```python
from build123d import *

# Parameters (mm, degrees)
SKETCH1_R           = 40.564550707
BOSS_EXTRUDE1_DEPTH = 10
BOSS_EXTRUDE2_DEPTH = 5.38
SKETCH5_R           = 76.2
BOSS_EXTRUDE3_DEPTH = 5.583348686
BOSS_EXTRUDE4_START = 9.66
SKETCH5_2_R         = 76.2
BOSS_EXTRUDE4_DEPTH = 9.66


with BuildPart() as part:
    # Sketch1 → Boss-Extrude1 (new body)
    with BuildSketch(Plane.XY):
        Circle(SKETCH1_R)
    extrude(amount=BOSS_EXTRUDE1_DEPTH)

    # Sketch2 → Boss-Extrude2 (add)
    with BuildSketch(Plane(origin=(0, 0, 0), x_dir=(-1, 0, 0), z_dir=(0, 0, -1))):
        with BuildLine():
            ThreePointArc((18.605098838, 17.572080057), (25.140246466, 15.180270653), (24.214003726, 8.283098686))
            ThreePointArc((24.214003726, 8.283098686), (25.586626057, 0.502262214), (24.520417146, -7.326448205))
            ThreePointArc((24.520417146, -7.326448205), (25.716623254, -14.181956771), (19.280375747, -16.828393011))
            ThreePointArc((19.280375747, -16.828393011), (13.228284865, -21.907537055), (5.915318308, -24.898528262))
            ThreePointArc((5.915318308, -24.898528262), (0.576376788, -29.362227423), (-4.933627979, -25.111491697))
            ThreePointArc((-4.933627979, -25.111491697), (-12.358341192, -22.409799269), (-18.605098838, -17.572080057))
            ThreePointArc((-18.605098838, -17.572080057), (-25.140246466, -15.180270653), (-24.214003726, -8.283098686))
            ThreePointArc((-24.214003726, -8.283098686), (-25.586626057, -0.502262214), (-24.520417146, 7.326448205))
            ThreePointArc((-24.520417146, 7.326448205), (-25.716623254, 14.181956771), (-19.280375747, 16.828393011))
            ThreePointArc((-19.280375747, 16.828393011), (-13.228284865, 21.907537055), (-5.915318308, 24.898528262))
            ThreePointArc((-5.915318308, 24.898528262), (-0.576376788, 29.362227423), (4.933627979, 25.111491697))
            ThreePointArc((4.933627979, 25.111491697), (12.358341192, 22.409799269), (18.605098838, 17.572080057))
        make_face()
    extrude(amount=BOSS_EXTRUDE2_DEPTH)

    # Sketch4 → Cut-Revolve2 (revolve, cut)
    with BuildSketch(Plane(origin=(0, 0, 0), x_dir=(0, 0, -1), z_dir=(0.9998069773781536, -0.01964708594067849, 0)), mode=Mode.PRIVATE) as cut_revolve2_sk:
        Polygon((0.153479633, 36.092584483), (0.153479633, 40.603125703), (-4.416651314, 40.603125703), (-4.416651314, 35.514398024), (-3.556, 32.394803966), (-3.556, 29.327755228), (0.657751111, 29.301116836), align=None)
    revolve(cut_revolve2_sk.sketch.rotate(Axis((0, 0, 95.775716375), (0, 0, -1)), 178.874232462), axis=Axis((0, 0, 95.775716375), (0, 0, -1)), mode=Mode.SUBTRACT)

    # Sketch5 → Boss-Extrude3 (add)
    with BuildSketch(Plane.XY.offset(10)):
        Circle(SKETCH5_R)
    extrude(amount=-BOSS_EXTRUDE3_DEPTH)

    # Sketch5<2> → Boss-Extrude4 (add)
    with BuildSketch(Plane.XY.offset(10).offset(BOSS_EXTRUDE4_START)):
        Circle(SKETCH5_2_R)
    extrude(amount=-BOSS_EXTRUDE4_DEPTH)


solid = part.part
```
Can you work these out from the model? Positions are in its coordinate system, mm. A direction names the side the tool comes from. Round coordinates to 2 decimals unless told otherwise and drop trailing zeros. Loops run counter-clockwise (first coordinate to the right, second up) from the corner with the lowest first, then second, coordinate; pieces in that order, holes last.
Item 1: Suppose I cut it at B-B, the plane x = 52. Write out the boundary of the cut face in (y, z), then the cut area to 3 significant figures.
Item 2: Suppose I cut it at C-C, the plane y = -51.5. Write out the boundary of the cut face in (x, z), then the cut area to 3 significant figures.
Item 3: Please list where these lines run through material, in increasing order: L1, parallel to Z at x = 11.5, y = -43; L2, parallel to X at y = -12, z = -0.75; L3, parallel to X at y = -16.5, z = 0.25.
Item 4: Suppose I cut it at A-A, the plane z = -2.5. Write out the boundary of the cut face in (x, y).
Item 5: Suppose I cut it at D-D, the plane z = 13.25. Write out the boundary of the cut face in (x, y), then the cut area to 3 significant figures.
Item 6: Which directions (+Z, -Z, +X, -X, +Y, -Y) give clear straight access to the entire face, cutting with the end or side of a thin tool? Please do faces 1 (the cylindrical face through (0.68, 29.36, -2.65)), 2 (the conical face through (28.62, 6.35, 1.42)), 3 (the cylindrical face through (-25.584, 0.613, -2.652)), 4 (the cylindrical face through (-0.68, -29.36, -2.65)).
Item 7: If we mould it in two halves opening along Y, with no side actions, what happens to faces 5 (the flat face through (-13, 24, 0)), 6 (the cylindrical face through (25.584, -0.613, -2.652)), 7 (the cylindrical face through (-25.085, 15.27, -2.652)), 8 (the conical face through (-32.27, 4.24, 3.6))? For each: +Y half, -Y half, draft (parallel to the pull), parting line (faces both ways), or undercut.
Item 8: Will these pins go through, and if not, where does the flat tip stop? pin 1 Ø1.5 at (x, z) = (-42.5, 5) entering from -Y; pin 2 Ø1.5 at (x, z) = (-26, 9.5) entering from +Y; pin 3 Ø8 at (x, y) = (-61, 38) entering from -Z.
Reported:
1. outline: (-55.7, 4.42) - (55.7, 4.42) - (55.7, 19.66) - (-55.7, 19.66) - close
1. area: 1,700 mm2
2. outline: (-56.16, 4.42) - (56.16, 4.42) - (56.16, 19.66) - (-56.16, 19.66) - close
2. area: 1,710 mm2
3. L1: z = 4.42 to 19.66
3. L2: x = -26.38 to 25.93
3. L3: x = -24.22 to 24.22
4. outline: (-24.52, -7.33) arc R5.56 ccw to (-19.28, -16.83) arc R25.59 ccw to (-5.92, -24.9) arc R5.56 ccw to (4.93, -25.11) arc R25.59 ccw to (18.61, -17.57) arc R5.56 ccw to (24.21, -8.28) arc R25.59 ccw to (24.52, 7.33) arc R5.56 ccw to (19.28, 16.83) arc R25.59 ccw to (5.92, 24.9) arc R5.56 ccw to (-4.93, 25.11) arc R25.59 ccw to (-18.61, 17.57) arc R5.56 ccw to (-24.21, 8.28) arc R25.59 ccw to start
5. outline: circle Ø152.4 at (0, 0)
5. area: 18,200 mm2
6. face 1: -Z, +Y
6. face 2: -Z
6. face 3: -Z, -X
6. face 4: -Z, -Y
7. face 5: draft
7. face 6: undercut
7. face 7: undercut
7. face 8: parting line
8. pin 1: stops at y = -63.74
8. pin 2: stops at y = 71.89
8. pin 3: stops at z = 4.42
